Geometry: see drawing. Coordinates: mm, zero at the bounding-box minimum. Coordinates: 2 decimals unless noted, no trailing zeros. Order: outer loops, then holes, each group sorted by start corner. A loop starts at its lowest first (then second) coordinate and runs counter-clockwise, first axis right, second up.
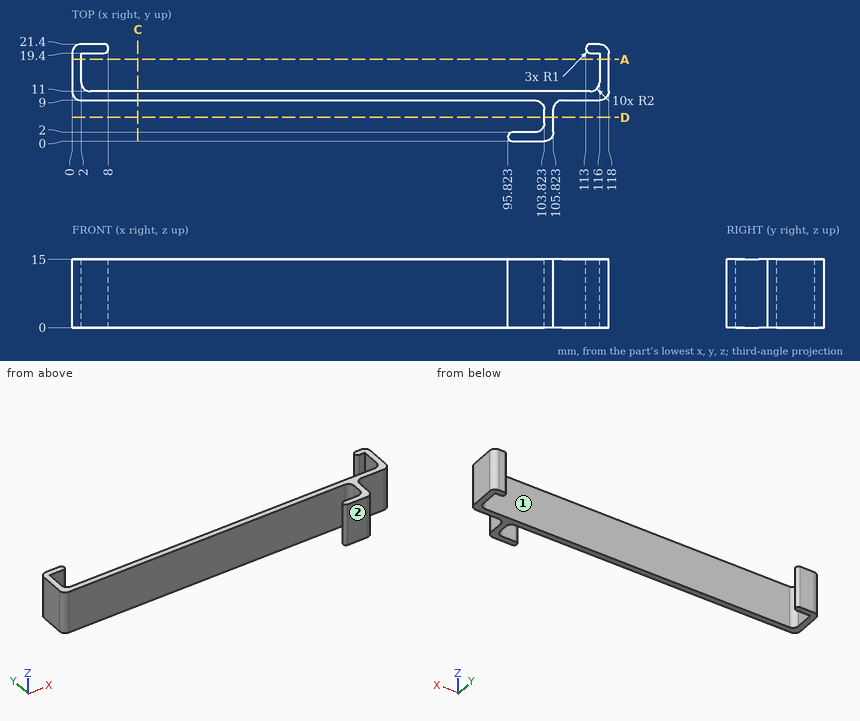
Item 1: Ray query, probe 1 along X at (y, z) = (19.25, 9.75); probe 2 along Y at (x, z) = (100, 4.5); probe 3 along X at (y, z) = (4.75, 10.5). Return the intervals inside material, ascending.
Response values:
probe 1: x = 0 to 2, 116 to 118
probe 2: y = 0 to 2, 9 to 11
probe 3: x = 103.82 to 105.82
Item 2: Draft query along X for the marked faces 1 and 2. Return one class per face: pulls with the +X half, pulls with the -X half, needs draft (parallel to the pull), parting line crosses it, or undercut.
Response values:
face 1: undercut
face 2: needs draft
Item 3: Pin query (flat end, axial travel): pin 1 Ø9 at (x, z) = (110, 11) entering from -Y; pin 2 Ø8 at (x, z) = (94.5, 12) entering from +Y; pin 3 Ø0.6 at (x, z) = (115.5, 10.5) entering from -Y. Return the tip coordinate at first contact, or that it passes through.
Response values:
pin 1: stops at y = 0.91
pin 2: stops at y = 11
pin 3: stops at y = 9
Item 4: Cut plane C-C on x = 14.5. Return loops of the section in (y, z), then the cut area to 3 significant figures.
Response values:
outline: (9, 0) - (11, 0) - (11, 15) - (9, 15) - close
area: 30.0 mm2
Item 5: Cut plane A-A on y = 18. Return loops of the section in (x, z), then the cut area to 3 significant figures.
Response values:
outline: (0, 0) - (2, 0) - (2, 15) - (0, 15) - close; (116, 0) - (118, 0) - (118, 15) - (116, 15) - close
area: 60.0 mm2
Item 6: Cut plane D-D on y = 5.25. Return loops of the section in (x, z).
Response values:
outline: (103.82, 0) - (105.82, 0) - (105.82, 15) - (103.82, 15) - close
